The listing builds one solid part. Answer for the finished solid, in the listing's coordinates (mm). Face numbers are marked on the shaded views. A direction names the side the tool comes from. Round coordinates to 2 decimals unless told otherwise and drop trailing zeros. Loops run counter-clockwise (first coordinate to the right, second up) from the corner with the lowest first, then second, coordinate; pieces in that order, holes last. Notation, with made-up numbers: (-23.5, 6.5) -> (-16.5, 6.5) arc R8 ccw to (-16.5, 20.5) -> close; hole circle Ø1 at (14.5, 37). An arc over 180 degrees is marked (long way). Write each question's results on one line, items separated by ' | '. Start each with the question number.
(1) Flat-ended cylindrical pins translate along their axes: pin 1 (2 mm diameter, centred on y = 10, z = -0.5, fed in from +X); pin 2 (3 mm diameter, centred on x = -5, y = 7.5, fed in from +Z); pin 3 (1 mm diameter, centred on y = 21, z = 1, fed in from -X). Find the tip coordinate at first contact, or state that the pin passes through.
(2) Straight lines are drawn through the part: probe 1 along Y at (x, z) = (1.75, 6.75); probe 2 along X at (y, z) = (26.5, 0); probe 3 along X at (y, z) = (18, 3.25). For each, find the intervals that lie inside material, in ascending order.
(3) The part is cut by section A-A (x = 0). Determine the outline of the cut face in (y, z).
(4) The part is cut by section B-B (y = 28.5). Determine the outline of the cut face in (x, z).
(5) For the marked faces 1 and 2, determine the directions among +Z, -Z, +X, -X, +Y, -Y from which every point of the face is accessible in a straight line to the end or side of a thin tool.
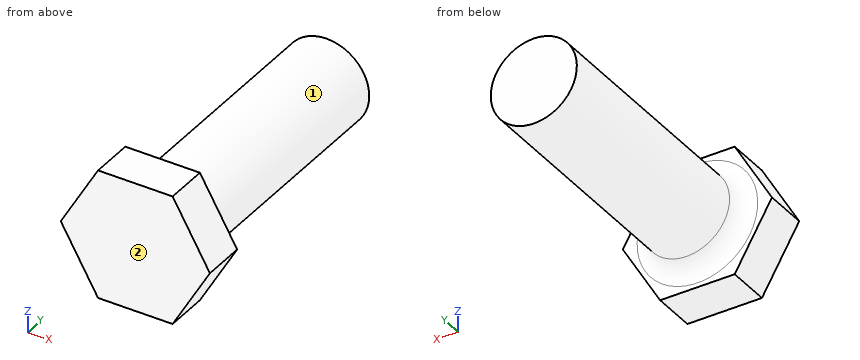
```python
from build123d import *

# Parameters (mm, degrees)
BOSS_EXTRUDE1_DEPTH = 5
SKETCH2_R           = 5
BOSS_EXTRUDE2_DEPTH = 30
FILLET1_R           = 2


with BuildPart() as part:
    # Sketch1 → Boss-Extrude1 (new body)
    with BuildSketch(Plane(origin=(0, 0, 0), x_dir=(1, 0, 0), z_dir=(0, 1, 0))):
        Polygon((8.660254038, 0), (4.330127019, 7.5), (-4.330127019, 7.5), (-8.660254038, 0), (-4.330127019, -7.5), (4.330127019, -7.5), align=None)
    extrude(amount=BOSS_EXTRUDE1_DEPTH)

    # Sketch2 → Boss-Extrude2 (add)
    with BuildSketch(Plane(origin=(0, 5, 0), x_dir=(1, 0, 0), z_dir=(0, 1, 0))):
        with Locations(Location((0, 0, 0), (0, 0, 270))):
            Circle(SKETCH2_R)
    extrude(amount=BOSS_EXTRUDE2_DEPTH)

    # Fillet1
    fillet1_edges = [part.edges().sort_by_distance(p)[0] for p in [
        (0, 5, -5),
    ]]
    fillet(fillet1_edges, radius=FILLET1_R)


solid = part.part
```
Checked values:
1) pin 1: stops at x = 5 | pin 2: stops at z = 3.57 | pin 3: stops at x = -4.97
2) probe 1: y = 0 to 5 | probe 2: x = -5 to 5 | probe 3: x = -3.8 to 3.8
3) outline: (0, -7.5) -> (5, -7.5) -> (5, -7) arc R2 cw to (7, -5) -> (35, -5) -> (35, 5) -> (7, 5) arc R2 cw to (5, 7) -> (5, 7.5) -> (0, 7.5) -> close
4) outline: circle Ø10 at (0, 0)
5) face 1: +Y | face 2: +Z, -Z, +X, -X, -Y
